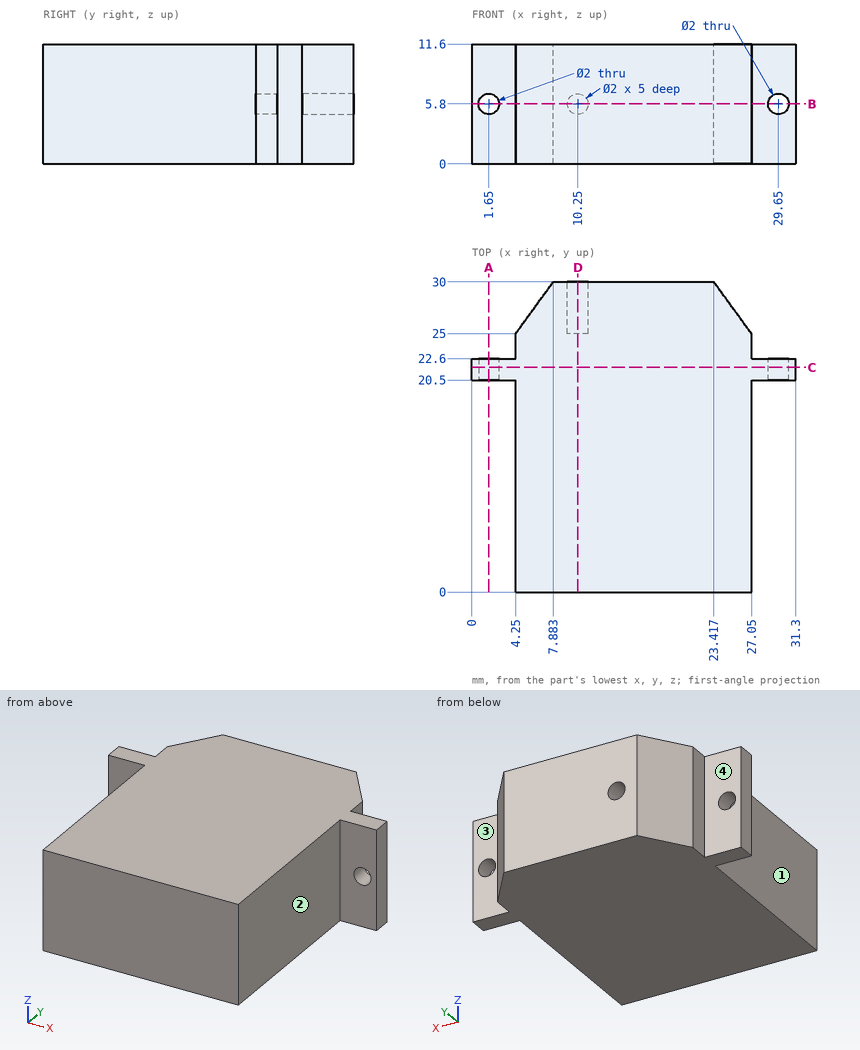
The figure shows three views and two pictorial views of one solid part (mm, origin at its lowest corner). Answer the questions. A direction names the side the tool comes from. Coordinates: 2 decimals unless noted, no trailing zeros. Loops run counter-clockwise (first coordinate to the right, second up) from the corner with the lowest first, then second, coordinate; pieces in that order, holes last. Notation, with made-up numbers: (37.25, 69) -> (56.25, 69) arc R15 ccw to (56.25, 73) -> close; hole circle Ø8 at (-25, 43.5). An arc over 180 degrees is marked (long way). Write item = value, one per line. Start each with the question number.
1) A cutting plane is placed at C-C (y = 21.75). Give the vertices of the cut face in (x, z).
2) Straight lines are drawn through the part: line 1 (Z direction, x = 29.65, y = 21.15); line 2 (X direction, y = 7.75, z = 5.25); line 3 (Y direction, x = 29, z = 3.5). For each, find the intervals that lie inside material, in ascending order. Write a range as from..to.
3) A tool of negligible diameter and unlimited length cuts with its end or side. For the marked faces 1, 2, 3 and 4, from which of +Z, -Z, +X, -X, +Y, -Y can it reach the whole face along a straight path? Write none if from no direction.
4) A cutting plane is placed at A-A (x = 1.65). Give the vertices of the cut face in (y, z).
5) A cutting plane is placed at D-D (x = 10.25). Give the vertices of the cut face in (y, z), then the cut area to 3 significant figures.
6) A cutting plane is placed at B-B (z = 5.8). Give the vertices of the cut face in (x, y), then the cut area to 3 significant figures.
7) Given pin 1 Ø2 at (x, z) = (29, 8) entering from -Y; pin 2 Ø2.5 at (y, z) = (24, 3) entering from -X; pin 3 Ø3.5 at (y, z) = (5, 6) entering from +X, each flat-ended and moving along its own axis, determine where each tip first touches the part or whether it passes through.
Responses:
q1.outline = (0, 0) -> (31.3, 0) -> (31.3, 11.6) -> (0, 11.6) -> close; hole circle Ø2 at (1.65, 5.8); hole circle Ø2 at (29.65, 5.8)
q2.line_1 = 0..4.8, 6.8..11.6
q2.line_2 = 4.25..27.05
q2.line_3 = 20.5..22.6
q3.face_1 = +Z, -Z, -X, -Y
q3.face_2 = +Z, -Z, +X, -Y
q3.face_3 = +Z, -Z, +X, +Y
q3.face_4 = +Z, -Z, -X, +Y
q4.outline = (20.5, 0) -> (22.6, 0) -> (22.6, 4.8) -> (20.5, 4.8) -> close; (20.5, 6.8) -> (22.6, 6.8) -> (22.6, 11.6) -> (20.5, 11.6) -> close
q5.outline = (0, 0) -> (30, 0) -> (30, 4.8) -> (25, 4.8) -> (25, 6.8) -> (30, 6.8) -> (30, 11.6) -> (0, 11.6) -> close
q5.area = 338 mm²
q6.outline = (0, 20.5) -> (0.65, 20.5) -> (0.65, 22.6) -> (0, 22.6) -> close; (2.65, 20.5) -> (4.25, 20.5) -> (4.25, 0) -> (27.05, 0) -> (27.05, 20.5) -> (28.65, 20.5) -> (28.65, 22.6) -> (27.05, 22.6) -> (27.05, 25) -> (23.42, 30) -> (11.25, 30) -> (11.25, 25) -> (9.25, 25) -> (9.25, 30) -> (7.88, 30) -> (4.25, 25) -> (4.25, 22.6) -> (2.65, 22.6) -> close; (30.65, 20.5) -> (31.3, 20.5) -> (31.3, 22.6) -> (30.65, 22.6) -> close
q6.area = 665 mm²
q7.pin_1 = 20.5
q7.pin_2 = 4.25
q7.pin_3 = 27.05
